Part print with two shaded views. Sizes in mm from the minimum x, y, z corner. A direction names the side the tool comes from. Give positions to 0.01 mm unless a question says otherwise; leave off trailing zeros. Order: outer loops, then holes, each group sorted by start corner. A loop starts at its lowest first (then second) coordinate and runs counter-clockwise, first axis right, second up. Notation, with made-up numbers: (36.25, 73) -> (75.25, 73) arc R16 cw to (75.25, 99) -> close; hole circle Ø10 at (-16, 72.5). An arc over 180 degrees is marked (long way). Answer in a Markdown table with one row per item. Add a question column.
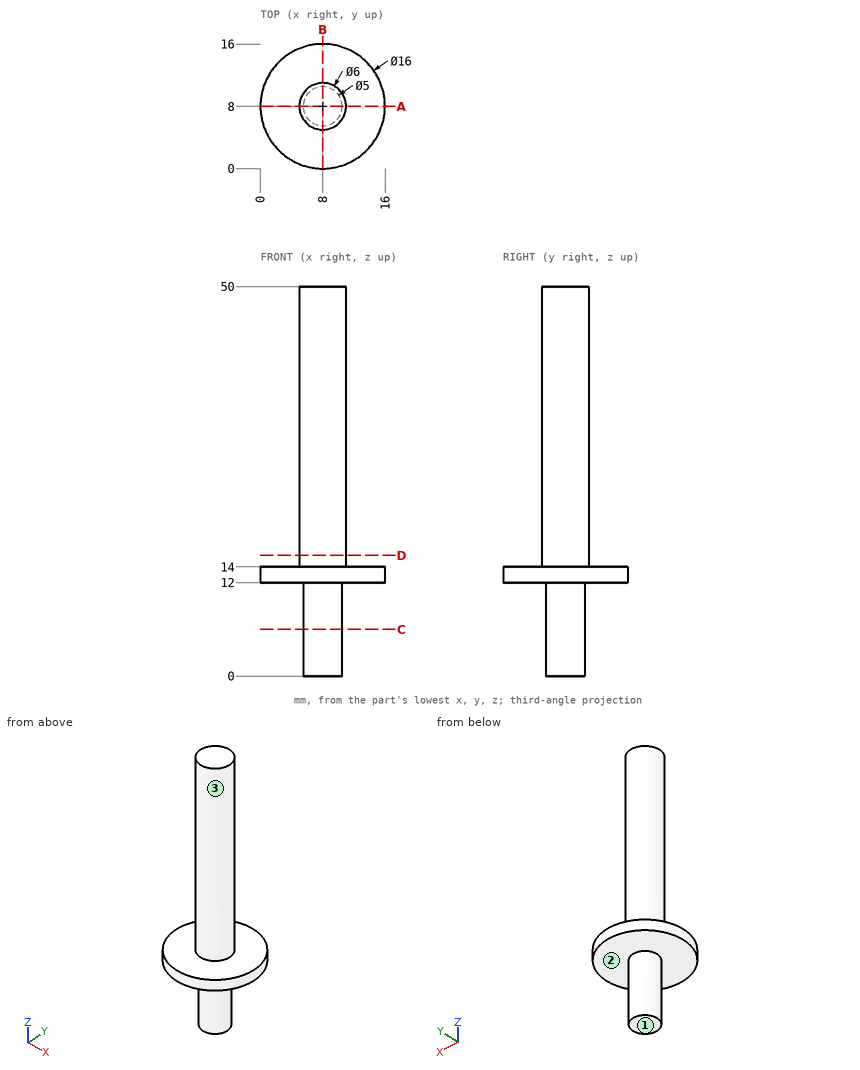
Item 1: Saw through at C-C on z = 6. List the corners of the cut face in (x, y), plus the area to 3 significant figures.
Item 2: Which spindle directions (+Z, -Z, +X, -X, +Y, -Y) get a long thin tool onto all of the face, cutting with end or side? Do the marked faces 1, 2 and 3. Say none if no direction does.
Item 3: Pin check, flat tips, straight feed: pin 1 Ø5 at (x, z) = (8, 38) entering from -Y; pin 2 Ø8 at (x, y) = (9, 11) entering from +Z; pin 3 Ø8 at (x, y) = (5, 14) entering from -Z; pin 4 Ø5 at (x, z) = (3.5, 16) entering from +Y. Stop position of each tip, or through.
Item 4: Saw through at D-D on z = 15.5. List the corners of the cut face in (x, y), plus the area to 3 significant figures.
Item 5: Saw through at A-A on y = 8. List the corners of the cut face in (x, z).
Item 6: Wall check: line 1 (Z direction, x = 2, y = 7.5); line 2 (X direction, y = 10, z = 32.5); line 3 (X direction, y = 5.25, z = 13). Give the ranges that are in metal, low to high.
Evaluation:
| question | item | result |
|---|---|---|
| 1 | outline | circle Ø5 at (8, 8) |
| 1 | area | 19.6 mm2 |
| 2 | face 1 | -Z, +X, -X, +Y, -Y |
| 2 | face 2 | -Z |
| 2 | face 3 | +Z |
| 3 | pin 1 | stops at y = 5 |
| 3 | pin 2 | stops at z = 50 |
| 3 | pin 3 | stops at z = 12 |
| 3 | pin 4 | stops at y = 15.42 |
| 4 | outline | circle Ø6 at (8, 8) |
| 4 | area | 28.3 mm2 |
| 5 | outline | (0, 12) -> (5.5, 12) -> (5.5, 0) -> (10.5, 0) -> (10.5, 12) -> (16, 12) -> (16, 14) -> (11, 14) -> (11, 50) -> (5, 50) -> (5, 14) -> (0, 14) -> close |
| 6 | line 1 | z = 12 to 14 |
| 6 | line 2 | x = 5.76 to 10.24 |
| 6 | line 3 | x = 0.49 to 15.51 |
